Could you check a few things on this drawing? It's one solid part, dimensions in mm from its lowest x, y, z. Round coordinates to 2 decimals unless told otherwise and drop trailing zeros. Write each loop counter-clockwise with the first axis right and the second up, starting at its lowest first coordinate (ties: lowest second). Pieces come first, ordered by that corner, then holes. Notation, with made-up numbers: (40, 0.5) -> (80, 0.5) arc R28 ccw to (80, 37.5) -> close; hole circle Ø9 at (60, -23). An arc over 180 degrees is marked (long way). Answer in a Markdown table with one row per item. Add a question column.
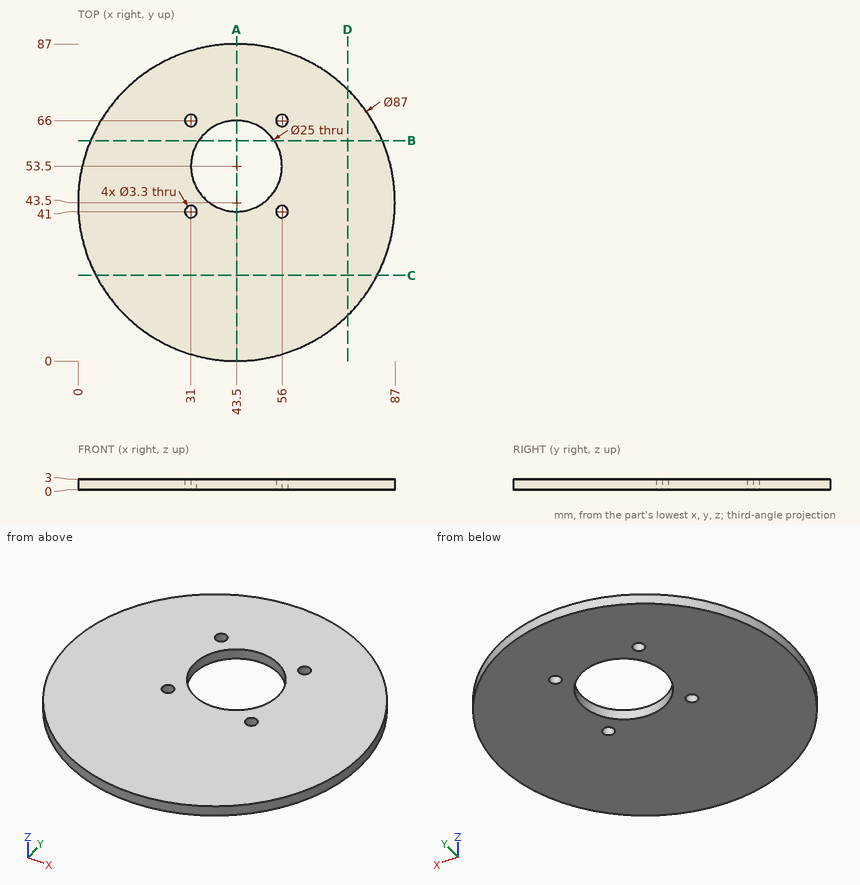
(1) Suppose I cut it at D-D, the plane x = 74. Please give me the cut outline in (y, z).
(2) I need wall thicknesses on L1, parallel to Y at x = 43.5, z = 1.05; L2, parallel to X at y = 39.5, z = 2; L3, parallel to X at y = 51, z = 1.3. Which ranges of each line are inside material? Lowest first, please.
(3) Suppose I cut it at C-C, the plane y = 23.5. Please give me the cut outline in (x, z).
(4) Suppose I cut it at A-A, the plane x = 43.5. Please give me the cut outline in (y, z).
(5) Suppose I cut it at B-B, the plane y = 60.5. Please give me the cut outline in (x, z), then the cut area to 3 significant figures.
(6) For P1, Ø2.5, axis at x = 56, y = 66, coming from the -Z side, with a flat end and sliding along its axis, tell me the tip position at first contact or that it passes through.
Response:
| question | item | result |
|---|---|---|
| 1 | outline | (12.48, 0) -> (74.52, 0) -> (74.52, 3) -> (12.48, 3) -> close |
| 2 | L1 | 0 to 41, 66 to 87 |
| 2 | L2 | 0.18 to 30.31, 31.69 to 55.31, 56.69 to 86.82 |
| 2 | L3 | 0.65 to 31.25, 55.75 to 86.35 |
| 3 | outline | (4.87, 0) -> (82.13, 0) -> (82.13, 3) -> (4.87, 3) -> close |
| 4 | outline | (0, 0) -> (41, 0) -> (41, 3) -> (0, 3) -> close; (66, 0) -> (87, 0) -> (87, 3) -> (66, 3) -> close |
| 5 | outline | (3.46, 0) -> (33.14, 0) -> (33.14, 3) -> (3.46, 3) -> close; (53.86, 0) -> (83.54, 0) -> (83.54, 3) -> (53.86, 3) -> close |
| 5 | area | 178 mm² |
| 6 | P1 | through |
